Geometry: final body of the model. Coordinates: model frame, mm. Coordinates: 2 decimals unless noted, no trailing zeros. Write each loop counter-clockwise with the first axis right and the second up, starting at its lowest first coordinate (ties: lowest second). Pieces come first, ordered by that corner, then holes. Notation, with made-up numbers: (-19.5, 5) -> (16.5, 5) arc R28 cw to (16.5, 27) -> close; hole circle Ø10 at (68.25, 18). An arc over 180 degrees is marked (long way). Answer as a JSON object with one key per item and string values. Group by question number.
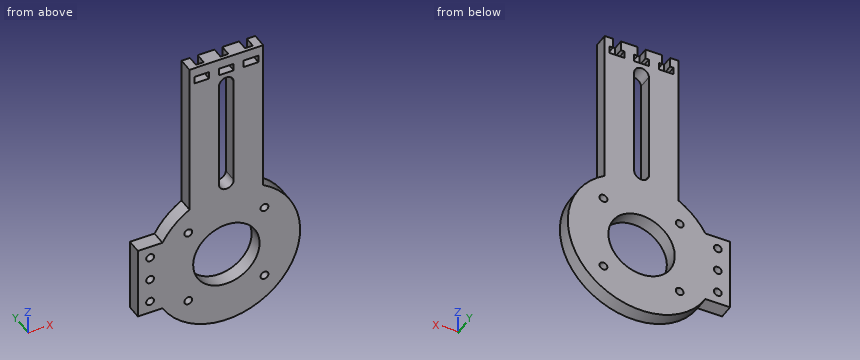
```python
from build123d import *

# Parameters (mm, degrees)
SKETCH_1_R          = 1.6
SKETCH_1_R_2        = 13.5
EXTRUDE_1_DEPTH     = 6
SKETCH_3_W          = 10
SKETCH_3_H          = 30
SKETCH_3_R          = 1.6
EXTRUDE_2_DEPTH     = 6
SKETCH_7_W          = 3.2
SKETCH_7_H          = 4
CUT_EXTRUDE_3_DEPTH = 14.5
SKETCH_8_W          = 6
SKETCH_8_H          = 3
CUT_EXTRUDE_4_DEPTH = 14.5
SKETCH_10_W         = 23.31764578
SKETCH_10_H         = 4
EXTRUDE_3_DEPTH     = 1.5
SKETCH_11_R         = 1.6
CUT_EXTRUDE_5_DEPTH = 10


with BuildPart() as part:
    # 草图1 → 凸台-拉伸1 (new body)
    with BuildSketch(Plane(origin=(0, 0, 0), x_dir=(1, 0, 0), z_dir=(0, 1, 0))):
        with BuildLine():
            Line((0, 64.019237886), (0, 0))
            Line((0, 0), (30, 0))
            Line((30, 0), (30, 64.019237886))
            ThreePointArc((30, 64.019237886), (15, 120), (0, 64.019237886))
        make_face()
        with BuildLine():
            ThreePointArc((12, 57.113903717), (15, 60.113903717), (18, 57.113903717))
            Line((18, 57.113903717), (18, 12.113903717))
            ThreePointArc((18, 12.113903717), (15, 9.113903717), (12, 12.113903717))
            Line((12, 12.113903717), (12, 57.113903717))
        make_face(mode=Mode.SUBTRACT)
        with Locations(Location((-0.5, 74.5, 0), (0, 0, 270))):
            Circle(SKETCH_1_R, mode=Mode.SUBTRACT)
        with Locations(Location((15, 90, 0), (0, 0, 270))):
            Circle(SKETCH_1_R_2, mode=Mode.SUBTRACT)
        with Locations(Location((30.5, 74.5, 0), (0, 0, 270))):
            Circle(SKETCH_1_R, mode=Mode.SUBTRACT)
        with Locations(Location((30.5, 105.5, 0), (0, 0, 270))):
            Circle(SKETCH_1_R, mode=Mode.SUBTRACT)
        with Locations(Location((-0.5, 105.5, 0), (0, 0, 270))):
            Circle(SKETCH_1_R, mode=Mode.SUBTRACT)
    extrude(amount=EXTRUDE_1_DEPTH)

    # 草图3 → 凸台-拉伸2 (add)
    with BuildSketch(Plane(origin=(0, 6, 0), x_dir=(1, 0, 0), z_dir=(0, 1, 0))):
        with Locations((-16, 90)):
            Rectangle(SKETCH_3_W, SKETCH_3_H)
        with Locations(Location((-16, 80, 0), (0, 0, 90))):
            Circle(SKETCH_3_R, mode=Mode.SUBTRACT)
        with Locations((-16, 90)):
            Circle(SKETCH_3_R, mode=Mode.SUBTRACT)
        with Locations(Location((-16, 100, 0), (0, 0, 90))):
            Circle(SKETCH_3_R, mode=Mode.SUBTRACT)
    extrude(amount=-EXTRUDE_2_DEPTH)

    # 草图7 → 切除-拉伸3 (cut)
    with BuildSketch(Plane.XZ):
        with Locations((25, -2)):
            Rectangle(SKETCH_7_W, SKETCH_7_H)
        with Locations((15, -2)):
            Rectangle(SKETCH_7_W, SKETCH_7_H)
        with Locations((5, -2)):
            Rectangle(SKETCH_7_W, SKETCH_7_H)
    extrude(amount=-CUT_EXTRUDE_3_DEPTH, mode=Mode.SUBTRACT)

    # 草图8 → 切除-拉伸4 (cut)
    with BuildSketch(Plane.XZ):
        with Locations((5, -5.5)):
            Rectangle(SKETCH_8_W, SKETCH_8_H)
        with Locations((15, -5.5)):
            Rectangle(SKETCH_8_W, SKETCH_8_H)
        with Locations((25, -5.5)):
            Rectangle(SKETCH_8_W, SKETCH_8_H)
    extrude(amount=-CUT_EXTRUDE_4_DEPTH, mode=Mode.SUBTRACT)

    # 草图10 → 凸台-拉伸3 (add)
    with BuildSketch(Plane.XZ):
        with Locations((15.05882289, -2)):
            Rectangle(SKETCH_10_W, SKETCH_10_H)
    extrude(amount=-EXTRUDE_3_DEPTH)

    # 草图11 → 切除-拉伸5 (cut)
    with BuildSketch(Plane(origin=(0, 6, 0), x_dir=(1, 0, 0), z_dir=(0, 1, 0))):
        with Locations(Location((-16, 90, 0), (0, 0, 90))):
            Circle(SKETCH_11_R)
    extrude(amount=-CUT_EXTRUDE_5_DEPTH, mode=Mode.SUBTRACT)


solid = part.part
```
Item 1: Section D-D on y = 3.1. Give the number of separate pieces and of enclosed holes in the cut face, then the cut area to 3 significant figures.
Item 2: Section A-A on z = -90. Output: boundary loops of the cut face in (x, y).
Item 3: Section B-B on z = -38. Output: boundary loops of the cut face in (x, y), then the cut area to 3 significant figures.
Item 4: Section C-C on x = -8. Output: boundary loops of the cut face in (y, z).
Item 5: Ray query, L1, parallel to Z at x = -16, y = 3.05; L2, parallel to X at y = 3.4, z = -90; L3, parallel to Z at x = 17.5, y = 2.2. Return the intervals inside material, ascending. Write a range as [from, to].
Item 6: Contact query for flat-ended pins moving along their axis: pin 1 (3 mm diameter, centred on x = -16, z = -90, fed in from -Y); pin 2 (1.8 mm diameter, centred on y = 3.5, z = -33.5, fed in from +X); pin 3 (0.9 mm diameter, centred on y = 3, z = -5, fed in from -X); pin 4 (3 mm diameter, centred on y = 2.5, z = -72.5, fed in from -X). Output: stop coordinate, or through.
Answer sheet:
{
 "1": {"separate pieces": "1", "enclosed holes": "9", "area": "3,870 mm^2"},
 "2": {"outline": "(-21, 0) -> (-17.6, 0) -> (-17.6, 6) -> (-21, 6) -> close; (-14.4, 0) -> (1.5, 0) -> (1.5, 6) -> (-14.4, 6) -> close; (28.5, 0) -> (45, 0) -> (45, 6) -> (28.5, 6) -> close"},
 "3": {"outline": "(0, 0) -> (12, 0) -> (12, 6) -> (0, 6) -> close; (18, 0) -> (30, 0) -> (30, 6) -> (18, 6) -> close", "area": "144 mm^2"},
 "4": {"outline": "(0, -109.26) -> (6, -109.26) -> (6, -70.74) -> (0, -70.74) -> close"},
 "5": {"L1": "z = [-105, -101.6], [-98.4, -91.6], [-88.4, -81.6], [-78.4, -75]", "L2": "x = [-21, -17.6], [-14.4, 1.5], [28.5, 45]", "L3": "z = [-119.9, -103.27], [-76.73, -58.77], [-10.46, -7], [-4, 0]"},
 "6": {"pin 1": "passes through", "pin 2": "stops at x = 30", "pin 3": "stops at x = 0", "pin 4": "stops at x = -10.38"}
}
